```python
from build123d import *

# Parameters (mm, degrees)
SKETCH1_R                      = 17
BOSS_EXTRUDE1_DEPTH            = 1.05
SKETCH2_W                      = 0.5
SKETCH2_H                      = 2
POLES_DEPTH                    = 1.2
POLES_DEPTH_BACK               = 7.3
SKETCH3_R                      = 1.5
BOSS_EXTRUDE3_DEPTH            = 1.2
SKETCH5_R                      = 17
BOSS_EXTRUDE5_DEPTH            = 26.5
SKETCH6_R                      = 18.5
REDUCTUR_DEPTH                 = 21.5
SKETCH35_R                     = 18.5
ENDPLATE_DEPTH                 = 1.5
SKETCH36_R                     = 6
BOSS_EXTRUDE25_DEPTH           = 6
F_3_1_3_1_DIAMETER_HOLE1_D     = 6
F_3_1_3_1_DIAMETER_HOLE1_DEPTH = 2.2
F_2_0_2_DIAMETER_HOLE1_D       = 2
F_2_0_2_DIAMETER_HOLE1_DEPTH   = 2.25
F_3_0MM_1_D                    = 3
F_3_0MM_1_DEPTH                = 7.5
F_3_0MM_1_TIP                  = 0.901290929
SKETCH_1_R                     = 3
EXTRUDE_1_DEPTH                = 21


with BuildPart() as part:
    # Sketch1 → Boss-Extrude1 (new body)
    with BuildSketch(Plane(origin=(41.25, 0, 0), x_dir=(0, 0, -1), z_dir=(1, 0, 0))):
        Circle(SKETCH1_R)
    extrude(amount=-BOSS_EXTRUDE1_DEPTH)

    # Sketch2 → Poles (add, two sides)
    with BuildSketch(Plane.ZY.offset(-40.2)) as poles_sk:
        with Locations((15.5, 0)):
            Rectangle(SKETCH2_W, SKETCH2_H)
        with Locations((-15.5, 0)):
            Rectangle(SKETCH2_W, SKETCH2_H)
    extrude(amount=POLES_DEPTH)
    extrude(poles_sk.sketch, amount=-POLES_DEPTH_BACK)

    # Sketch3 → Boss-Extrude3 (add)
    with BuildSketch(Plane.ZY.offset(-40.2)):
        Circle(SKETCH3_R)
    extrude(amount=BOSS_EXTRUDE3_DEPTH)

    # Sketch5 → Boss-Extrude5 (add)
    with BuildSketch(Plane(origin=(39, 0, 0), x_dir=(0, 0, -1), z_dir=(1, 0, 0))):
        Circle(SKETCH5_R)
    extrude(amount=-BOSS_EXTRUDE5_DEPTH)

    # Sketch6 → Reductur (add)
    with BuildSketch(Plane(origin=(12.5, 0, 0), x_dir=(0, 0, -1), z_dir=(1, 0, 0))):
        Circle(SKETCH6_R)
    extrude(amount=-REDUCTUR_DEPTH)

    # Sketch35 → Endplate (add)
    with BuildSketch(Plane.ZY.offset(9)):
        Circle(SKETCH35_R)
    extrude(amount=ENDPLATE_DEPTH)

    # Sketch36 → Boss-Extrude25 (add)
    with BuildSketch(Plane.ZY.offset(10.5)):
        with Locations((0, 7)):
            Circle(SKETCH36_R)
    extrude(amount=BOSS_EXTRUDE25_DEPTH)

    # Ø3.1 (3.1) Diameter Hole1
    with Locations(Plane.ZY.offset(16.5)):
        with Locations((0, 7)):
            Hole(F_3_1_3_1_DIAMETER_HOLE1_D / 2, depth=F_3_1_3_1_DIAMETER_HOLE1_DEPTH)

    # Ø2.0 (2) Diameter Hole1
    with Locations(Plane(origin=(41.25, 0, 0), x_dir=(0, 0, -1), z_dir=(1, 0, 0))):
        with Locations((0, 0)):
            Hole(F_2_0_2_DIAMETER_HOLE1_D / 2, depth=F_2_0_2_DIAMETER_HOLE1_DEPTH)

    # Ø3.0mm 定位孔1
    with Locations(Plane(origin=(-10.5, 0, -15.5), x_dir=(0, 0, -1), z_dir=(-1, 0, 0))):
        with Locations((0, 0), (-7.75, -13.423393759), (-23.50507477, -13.272858695), (-31, 0), (-23.25, 13.423393759), (-7.75, 13.423393759)):
            Hole(F_3_0MM_1_D / 2, depth=F_3_0MM_1_DEPTH)
            with Locations((0, 0, -(F_3_0MM_1_DEPTH + F_3_0MM_1_TIP / 2))):  # 118° drill point
                Cone(0, F_3_0MM_1_D / 2, F_3_0MM_1_TIP, mode=Mode.SUBTRACT)

    # 草圖1 → 填料-伸長1 (add)
    with BuildSketch(Plane.ZY.offset(10.5)):
        with Locations((0, 7)):
            Circle(SKETCH_1_R)
    extrude(amount=EXTRUDE_1_DEPTH)


solid = part.part
```
Work out the finished part from the listing and answer in its coordinate system (mm). A direction names the side the tool comes from. Give positions to 0.01 mm unless a question says otherwise; leave off trailing zeros. Order: outer loops, then holes, each group sorted by start corner. A loop starts at its lowest first (then second) coordinate and runs counter-clockwise, first axis right, second up. Notation, with made-up numbers: (13, -31.5) - (18, -31.5) arc R29 ccw to (18, 2.5) - close; hole circle Ø5 at (-35.75, -35). An arc over 180 degrees is marked (long way). One line per item, written item: value. Start each with the question number.
1. Which of the six approach directions +Z, -Z, +X, -X, +Y, -Y give full straight-line access (tool end or side, diameter ignored) to faces 1 (the face through (44, 0, -15.75)), 2 (the face through (39.61, 0.07, -1.5)), 3 (the face through (44, 0, -15.25)), 4 (the face through (-6.7, -11.96, -8.08)), 5 (the face through (40, -1, 0))?
2. Section B-B, the plane z = 5 is taken. Write down the section's boundary in (x, y).
3. Each of these flat-tipped pins is pushed along its axis until it touches: pin 1 Ø0.6 at (x, z) = (43, 15.5) entering from +Y; pin 2 Ø10 at (y, z) = (-8.5, 14) entering from +X; pin 3 Ø2 at (y, z) = (-9, 7.5) entering from -X. Where does it stop, or does it pass through?
4. For a pull along Y with two mould halves and no side action, classify faces 6 (the face through (-24, 7, -3)), 7 (the face through (-2.255, -13.682, 7.784)), 8 (the face through (-16.5, 10, 1)) as released by +Y, released by -Y, zero draft, split by the parting line, or undercut.
5. Section C-C, the plane x = -7 is taken. Write down the section's boundary in (y, z), then the cut area to 3 significant figures.
6. Consider line 1 (X direction, y = 7, z = -9); line 2 (Y direction, x = -7.5, z = -7.75); line 3 (X direction, y = 6, z = 0). Determine where each line is inside the solid, lowest interval first.
7. Section D-D, the plane x = 1 is taken. Write down the section's boundary in (y, z), then the cut area to 3 significant figures.
8. Section A-A, the plane y = 7 is taken. Write down the section's boundary in (x, z), then the cut area to 3 significant figures.
Filled sheet:
1. face 1: -Z, +X, +Y, -Y
1. face 2: none
1. face 3: +X, +Y, -Y
1. face 4: -X
1. face 5: +X
2. outline: (-16.5, 3.68) - (-10.5, 3.68) - (-10.5, -17.81) - (12.5, -17.81) - (12.5, -16.25) - (39, -16.25) - (39, 16.25) - (12.5, 16.25) - (12.5, 17.81) - (-10.5, 17.81) - (-10.5, 10.32) - (-16.5, 10.32) - close; (40.2, -16.25) - (41.25, -16.25) - (41.25, 16.25) - (40.2, 16.25) - close
3. pin 1: y = 1
3. pin 2: x = 41.25
3. pin 3: x = -10.5
4. face 6: split by the parting line
4. face 7: undercut
4. face 8: zero draft
5. outline: circle Ø37 at (0, 0); hole circle Ø3 at (-13.42, -7.75); hole circle Ø3 at (-13.42, 7.75); hole circle Ø3 at (0, -15.5); hole circle Ø3 at (0, 15.5); hole circle Ø3 at (13.27, 8.01); hole circle Ø3 at (13.42, -7.75)
5. area: 1,030 mm²
6. line 1: -10.5 to 39, 40.2 to 41.25
6. line 2: -16.8 to -14.92, -11.92 to 11.92, 14.92 to 16.8
6. line 3: -31.5 to 39, 40.2 to 41.25
7. outline: circle Ø37 at (0, 0)
7. area: 1,080 mm²
8. outline: (-31.5, -3) - (-16.5, -3) - (-16.5, -6) - (-10.5, -6) - (-10.5, -17.12) - (12.5, -17.12) - (12.5, -15.49) - (39, -15.49) - (39, 15.49) - (12.5, 15.49) - (12.5, 17.12) - (-10.5, 17.12) - (-10.5, 6) - (-16.5, 6) - (-16.5, 3) - (-31.5, 3) - close; (40.2, -15.49) - (41.25, -15.49) - (41.25, 15.49) - (40.2, 15.49) - close
8. area: 1,800 mm²
